```python
from build123d import *

# Parameters (mm, degrees)
BOSS_EXTRUDE1_DEPTH       = 66
M3X0_5_TAPPED_HOLE1_D     = 2.5
M3X0_5_TAPPED_HOLE1_DEPTH = 7.5
M3X0_5_TAPPED_HOLE1_TIP   = 0.751075774
M2X0_4_TAPPED_HOLE1_D     = 1.6
M2X0_4_TAPPED_HOLE1_DEPTH = 5.2
M2X0_4_TAPPED_HOLE1_TIP   = 0.480688495
M3X0_5_TAPPED_HOLE2_D     = 2.5
M3X0_5_TAPPED_HOLE2_DEPTH = 7.5
M3X0_5_TAPPED_HOLE2_TIP   = 0.751075774
M2X0_4_TAPPED_HOLE2_D     = 1.6
M2X0_4_TAPPED_HOLE2_DEPTH = 5.2
M2X0_4_TAPPED_HOLE2_TIP   = 0.480688495
CUT_EXTRUDE1_DEPTH        = 67.749502158


with BuildPart() as part:
    # Sketch1 → Boss-Extrude1 (new body)
    with BuildSketch(Plane(origin=(0, 66, 0), x_dir=(1, 0, 0), z_dir=(0, 1, 0))):
        Polygon((3.829824533, 1.282917234), (-5.180847956, -5.026423564), (-5.180847956, -9.026423564), (0.819152044, -9.026423564), (0.819152044, -5.026423564), (5.479158688, -0.366416921), align=None)
    extrude(amount=-BOSS_EXTRUDE1_DEPTH)

    # M3x0.5 Tapped Hole1
    with Locations(Plane(origin=(0, 0, 0), x_dir=(-1, 0, 0), z_dir=(0, -1, 0))):
        with Locations((2.180847956, -6.526423564)):
            Hole(M3X0_5_TAPPED_HOLE1_D / 2, depth=M3X0_5_TAPPED_HOLE1_DEPTH)
            with Locations((0, 0, -(M3X0_5_TAPPED_HOLE1_DEPTH + M3X0_5_TAPPED_HOLE1_TIP / 2))):  # 118° drill point
                Cone(0, M3X0_5_TAPPED_HOLE1_D / 2, M3X0_5_TAPPED_HOLE1_TIP, mode=Mode.SUBTRACT)

    # M2x0.4 Tapped Hole1
    with Locations(Plane(origin=(0, 0, 0), x_dir=(-1, 0, 0), z_dir=(0, -1, 0))):
        with Locations((-0.219152044, -3.326423564)):
            Hole(M2X0_4_TAPPED_HOLE1_D / 2, depth=M2X0_4_TAPPED_HOLE1_DEPTH)
            with Locations((0, 0, -(M2X0_4_TAPPED_HOLE1_DEPTH + M2X0_4_TAPPED_HOLE1_TIP / 2))):  # 118° drill point
                Cone(0, M2X0_4_TAPPED_HOLE1_D / 2, M2X0_4_TAPPED_HOLE1_TIP, mode=Mode.SUBTRACT)

    # M3x0.5 Tapped Hole2
    with Locations(Plane(origin=(-2.180847956, 66, 6.526423564), x_dir=(0, 0, 1), z_dir=(0, 1, 0))):
        with Locations((0, 0)):
            Hole(M3X0_5_TAPPED_HOLE2_D / 2, depth=M3X0_5_TAPPED_HOLE2_DEPTH)
            with Locations((0, 0, -(M3X0_5_TAPPED_HOLE2_DEPTH + M3X0_5_TAPPED_HOLE2_TIP / 2))):  # 118° drill point
                Cone(0, M3X0_5_TAPPED_HOLE2_D / 2, M3X0_5_TAPPED_HOLE2_TIP, mode=Mode.SUBTRACT)

    # M2x0.4 Tapped Hole2
    with Locations(Plane(origin=(0.219152044, 66, 3.326423564), x_dir=(0, 0, 1), z_dir=(0, 1, 0))):
        with Locations((0, 0)):
            Hole(M2X0_4_TAPPED_HOLE2_D / 2, depth=M2X0_4_TAPPED_HOLE2_DEPTH)
            with Locations((0, 0, -(M2X0_4_TAPPED_HOLE2_DEPTH + M2X0_4_TAPPED_HOLE2_TIP / 2))):  # 118° drill point
                Cone(0, M2X0_4_TAPPED_HOLE2_D / 2, M2X0_4_TAPPED_HOLE2_TIP, mode=Mode.SUBTRACT)

    # Sketch12 → Cut-Extrude1 (cut, through all)
    with BuildSketch(Plane(origin=(0.657199769, 0, 0.938578541), x_dir=(-0.8191520444364442, 0, 0.5735764361404623), z_dir=(-0.5735764361404623, 0, -0.8191520444364442))):
        with BuildLine():
            Line((-1.325998276, 44.400000009), (1.174001724, 44.400000009))
            ThreePointArc((1.174001724, 44.400000009), (2.774001716, 46.000000001), (1.174001724, 47.599999993))
            Line((1.174001724, 47.599999993), (-1.325998276, 47.599999993))
            ThreePointArc((-1.325998276, 47.599999993), (-2.925998268, 46.000000001), (-1.325998276, 44.400000009))
        make_face()
        with BuildLine():
            Line((-1.325998276, 18.400000007), (1.174001724, 18.400000007))
            ThreePointArc((1.174001724, 18.400000007), (2.774001716, 19.999999999), (1.174001724, 21.599999991))
            Line((1.174001724, 21.599999991), (-1.325998276, 21.599999991))
            ThreePointArc((-1.325998276, 21.599999991), (-2.925998268, 19.999999999), (-1.325998276, 18.400000007))
        make_face()
    extrude(amount=-CUT_EXTRUDE1_DEPTH, mode=Mode.SUBTRACT)


solid = part.part
```
Geometry check sheet. Reference: the model listing, model coordinates, mm. A direction names the side the tool comes from. Coordinates: 2 decimals unless noted, no trailing zeros. Order: outer loops, then holes, each group sorted by start corner. A loop starts at its lowest first (then second) coordinate and runs counter-clockwise, first axis right, second up. Notation, with made-up numbers: (-15, 39.5) - (31, 39.5) arc R25 ccw to (31, 51.5) - close; hole circle Ø5 at (42.25, 34.25). An arc over 180 degrees is marked (long way). Use one line per item in the form item = value.
1. Section check A-A (y = 46.5). Record the boundary of the cut face in (x, z), then the cut area to 3 significant figures.
Here are the results:
outline = (-5.18, 5.03) - (-1.55, 2.48) - (0.82, 5.87) - (0.82, 9.03) - (-5.18, 9.03) - close; (2.99, -0.69) - (3.83, -1.28) - (5.48, 0.37) - (4.45, 1.39) - close
area = 33.6 mm²
2. Section check B-B (y = 27). Record the boundary of the cut face in (x, z).
Here are the results:
outline = (-5.18, 5.03) - (3.83, -1.28) - (5.48, 0.37) - (0.82, 5.03) - (0.82, 9.03) - (-5.18, 9.03) - close
3. Gauge pin test, flat ends, axial feed: pin 1 (1.3 mm diameter, centred on x = 0.22, z = 3.33, fed in from +Y); pin 2 (4 mm diameter, centred on x = 1.5, z = 2, fed in from -Y); pin 3 (4.5 mm diameter, centred on y = 41.5, z = 8, fed in from +X); pin 4 (1.5 mm diameter, centred on x = -2.18, z = 6.53, fed in from -Y). Record the tip position at first contact, or that the pin passes through.
Here are the results:
pin_1 = 60.71
pin_2 = 0
pin_3 = 0.82
pin_4 = 7.8
4. Draft check along Z on faces 6 (the face through (0.09, 5.6, 3.28)), 7 (the face through (2, 21.6, 2)), 8 (the face through (-0.657, 19.965, 3.897)). Enter one of: pulls with the +Z half, pulls with the -Z half, needs draft (parallel to the pull), parting line crosses it, or undercut.
Here are the results:
face_6 = undercut
face_7 = needs draft
face_8 = pulls with the -Z half
5. Scan lines: line 1 (Y direction, x = 0.25, z = 2.25); line 2 (Y direction, x = 0.25, z = 3.25); line 3 (X direction, y = 16.5, z = 5.25). Record each from-to range of solid material in increasing order.
Here are the results:
line_1 = 0 to 18.4, 21.6 to 44.4, 47.6 to 66
line_2 = 5.63 to 18.48, 21.52 to 44.48, 47.52 to 60.37
line_3 = -5.18 to 0.82
6. Access from +Z, -Z, +X, -X, +Y, -Y to the whole of each face (thin tool, end or side, straight path). Record for faces 1 (the face through (-0.27, 63.36, 3.96)), 2 (the face through (0.115, 2.636, 2.533)), 3 (the face through (0.819, 33, 7)), 4 (the face through (2, 18.4, 2)), 5 (the face through (-0.612, 33.462, 1.828)).
Here are the results:
face_1 = +Y
face_2 = -Y
face_3 = +Z, +X, +Y, -Y
face_4 = none
face_5 = -Z, -X, +Y, -Y
